Source: CAD feature listing. Evaluate the final solid. Frame: model axes, mm. A direction names the side the tool comes from. Give positions to 0.01 mm unless a question says otherwise; leave off trailing zeros. Order: outer loops, then holes, each group sorted by start corner. A loop starts at its lowest first (then second) coordinate and runs counter-clockwise, first axis right, second up.
```python
from build123d import *

# Parameters (mm, degrees)
F0_W      = 76.2
F0_H      = 76.2
F1_DEPTH  = 38.1
F2_W      = 11.73516
F2_H      = 2.54
F3_DEPTH  = 1.27
F5_DEPTH  = 1.27
F7_DEPTH  = 1.27
F9_DEPTH  = 1.27
F11_DEPTH = 1.27
F13_DEPTH = 1.27
F14_R     = 1.27


with BuildPart() as f1:
    # F0 (on Top) → F1 (new body, symmetric)
    with BuildSketch(Plane.XY):
        Rectangle(F0_W, F0_H)
    extrude(amount=F1_DEPTH, both=True)

    # F2 (on face) → F3 (cut, symmetric)
    with BuildSketch(Plane.XZ.offset(38.1)):
        with Locations((-7.13758, 21.63039)):
            Rectangle(F2_W, F2_H)
        Polygon((0, 22.90039), (-1.27, 22.90039), (-1.27, 20.36039), (0, 20.36039), (1.27, 20.36039), (1.27, 22.90039), align=None)
        Polygon((0, 20.36039), (-1.27, 20.36039), (-1.27, 0), (-1.27, -22.90039), (0, -22.90039), (1.27, -22.90039), (1.27, 0), (1.27, 20.36039), align=None)
        with Locations((7.13758, 21.63039)):
            Rectangle(F2_W, F2_H)
        Polygon((0, -22.90039), (-1.27, -22.90039), (-13.00516, -22.90039), (-13.00516, -25.44039), (0, -25.44039), (13.00516, -25.44039), (13.00516, -22.90039), (1.27, -22.90039), align=None)
    extrude(amount=F3_DEPTH, both=True, mode=Mode.SUBTRACT)

    # F4 (on face) → F5 (cut, symmetric)
    with BuildSketch(Plane(origin=(0, 38.1, 0), x_dir=(-1, 0, 0), z_dir=(0, 1, 0))):
        Polygon((5.588, 26.286197), (5.588, 23.746197), (10.960088, 23.746197), (12.230088, 23.746197), (13.500088, 23.746197), (19.957788, 23.746197), (19.957788, 26.286197), (12.230088, 26.286197), align=None)
        Polygon((12.230088, 23.746197), (10.960088, 23.746197), (10.960088, -21.1963), (12.230088, -21.1963), (13.500088, -21.1963), (13.500088, 23.746197), align=None)
        Polygon((12.230088, -21.1963), (10.960088, -21.1963), (5.588, -21.1963), (5.588, -23.7363), (12.230088, -23.7363), (19.957788, -23.7363), (19.957788, -21.1963), (13.500088, -21.1963), align=None)
        Polygon((-7.667548, 26.286197), (-14.804196, -10.425624), (-21.940843, 26.286197), (-24.528392, 26.286197), (-14.804196, -23.7363), (-5.08, 26.286197), align=None)
    extrude(amount=F5_DEPTH, both=True, mode=Mode.SUBTRACT)

    # F6 (on face) → F7 (cut, symmetric)
    with BuildSketch(Plane(origin=(-38.1, 0, 0), x_dir=(0, -1, 0), z_dir=(-1, 0, 0))):
        Polygon((-14.887291, 25.654), (0, -25.721655), (14.887291, 25.654), (12.2428, 25.654), (0, -16.595586), (-12.2428, 25.654), align=None)
    extrude(amount=F7_DEPTH, both=True, mode=Mode.SUBTRACT)

    # F8 (on face) → F9 (cut, symmetric)
    with BuildSketch(Plane.YZ.offset(38.1)):
        Polygon((-22.352, 27.513674), (-22.352, 24.973674), (-15.24, 24.973674), (-13.97, 24.973674), (-12.7, 24.973674), (-5.588, 24.973674), (-5.588, 27.513674), (-13.97, 27.513674), align=None)
        Polygon((-13.97, 24.973674), (-15.24, 24.973674), (-15.24, -26.48152), (-13.97, -26.48152), (-12.7, -26.48152), (-12.7, 24.973674), align=None)
        Polygon((-13.97, -26.48152), (-15.24, -26.48152), (-22.352, -26.48152), (-22.352, -29.02152), (-13.97, -29.02152), (-5.588, -29.02152), (-5.588, -26.48152), (-12.7, -26.48152), align=None)
        Polygon((13.97, 24.973674), (12.7, 24.973674), (12.7, -26.48152), (13.97, -26.48152), (15.24, -26.48152), (15.24, 24.973674), align=None)
        Polygon((5.588, 24.973674), (12.7, 24.973674), (13.97, 24.973674), (15.24, 24.973674), (22.352, 24.973674), (22.352, 27.513674), (13.97, 27.513674), (5.588, 27.513674), align=None)
        Polygon((13.97, -26.48152), (12.7, -26.48152), (5.588, -26.48152), (5.588, -29.02152), (13.97, -29.02152), (22.352, -29.02152), (22.352, -26.48152), (15.24, -26.48152), align=None)
    extrude(amount=F9_DEPTH, both=True, mode=Mode.SUBTRACT)

    # F10 (on face) → F11 (cut, symmetric)
    with BuildSketch(Plane(origin=(0, 0, -38.1), x_dir=(1, 0, 0), z_dir=(0, 0, -1))):
        Polygon((-22.352, 25.81735), (-22.352, 23.27735), (-15.24, 23.27735), (-13.97, 23.27735), (-12.7, 23.27735), (-5.588, 23.27735), (-5.588, 25.81735), (-13.97, 25.81735), align=None)
        Polygon((-13.97, 23.27735), (-15.24, 23.27735), (-15.24, -23.1902), (-13.97, -23.1902), (-12.7, -23.1902), (-12.7, 23.27735), align=None)
        Polygon((-13.97, -23.1902), (-15.24, -23.1902), (-22.352, -23.1902), (-22.352, -25.7302), (-13.97, -25.7302), (-5.588, -25.7302), (-5.588, -23.1902), (-12.7, -23.1902), align=None)
        Polygon((5.08, 25.81735), (16.829143, -25.7302), (28.578286, 25.81735), (25.973143, 25.81735), (16.829143, -14.300538), (7.685143, 25.81735), align=None)
    extrude(amount=F11_DEPTH, both=True, mode=Mode.SUBTRACT)

    # F12 (on face) → F13 (cut, symmetric)
    with BuildSketch(Plane.XY.offset(38.1)):
        Polygon((27.891114, -27.228153), (27.891114, -24.688153), (21.323074, -24.688153), (20.053074, -24.688153), (18.783074, -24.688153), (12.215033, -24.688153), (12.215033, -27.228153), (20.053074, -27.228153), align=None)
        Polygon((20.053074, -24.688153), (21.323074, -24.688153), (21.323074, 24.24637), (20.053074, 24.24637), (18.783074, 24.24637), (18.783074, -24.688153), align=None)
        Polygon((20.053074, 24.24637), (21.323074, 24.24637), (27.891114, 24.24637), (27.891114, 26.78637), (20.053074, 26.78637), (12.215033, 26.78637), (12.215033, 24.24637), (18.783074, 24.24637), align=None)
        Polygon((7.83804, -27.228153), (7.83804, -24.688153), (1.27, -24.688153), (0, -24.688153), (-1.27, -24.688153), (-7.83804, -24.688153), (-7.83804, -27.228153), (-0.004473, -27.228153), (0.004473, -27.228153), align=None)
        Polygon((0, -24.688153), (1.27, -24.688153), (1.27, 24.24637), (0, 24.24637), (-1.27, 24.24637), (-1.27, -24.688153), align=None)
        Polygon((0, 24.24637), (1.27, 24.24637), (7.83804, 24.24637), (7.83804, 26.78637), (0, 26.78637), (-7.83804, 26.78637), (-7.83804, 24.24637), (-1.27, 24.24637), align=None)
        Polygon((-20.053074, -27.228153), (-12.215033, -27.228153), (-12.215033, -24.688153), (-18.783074, -24.688153), (-20.053074, -24.688153), (-21.323074, -24.688153), (-27.891114, -24.688153), (-27.891114, -27.228153), align=None)
        Polygon((-20.053074, -24.688153), (-18.783074, -24.688153), (-18.783074, 24.24637), (-20.053074, 24.24637), (-21.323074, 24.24637), (-21.323074, -24.688153), align=None)
        Polygon((-20.053074, 24.24637), (-18.783074, 24.24637), (-12.215033, 24.24637), (-12.215033, 26.78637), (-20.053074, 26.78637), (-27.891114, 26.78637), (-27.891114, 24.24637), (-21.323074, 24.24637), align=None)
    extrude(amount=F13_DEPTH, both=True, mode=Mode.SUBTRACT)

    # F14
    f14_edges = [f1.edges().sort_by_distance(p)[0] for p in [
        (38.1, 0, 38.1),
        (0, -38.1, 38.1),
        (-38.1, 0, 38.1),
        (0, 38.1, 38.1),
        (-38.1, -38.1, 0),
        (0, -38.1, -38.1),
        (38.1, -38.1, 0),
        (-38.1, 0, -38.1),
        (-38.1, 38.1, 0),
        (38.1, 38.1, 0),
        (0, 38.1, -38.1),
        (38.1, 0, -38.1),
    ]]
    fillet(f14_edges, radius=F14_R)


solid = f1.part
```
1) Section query A-A, the plane x = 20. Return the cut outline in (y, z).
Report:
outline: (-38.1, -36.83) arc R1.27 ccw to (-36.83, -38.1) - (0.39, -38.1) - (0.39, -36.83) - (11.82, -36.83) - (11.82, -38.1) - (36.83, -38.1) arc R1.27 ccw to (38.1, -36.83) - (38.1, 2.99) - (36.83, 2.99) - (36.83, 16.3) - (38.1, 16.3) - (38.1, 36.83) arc R1.27 ccw to (36.83, 38.1) - (26.79, 38.1) - (26.79, 36.83) - (-27.23, 36.83) - (-27.23, 38.1) - (-36.83, 38.1) arc R1.27 ccw to (-38.1, 36.83) - close
2) Pin query (flat end, axial travel): pin 1 (1 mm diameter, centred on x = 37.5, z = -28, fed in from +Y); pin 2 (0.6 mm diameter, centred on x = -6, y = -37.5, fed in from +Z); pin 3 (1 mm diameter, centred on y = 1.5, z = 37.5, fed in from +X). Return the tip coordinate at first contact, or that it passes through.
Report:
pin 1: stops at y = 38.09
pin 2: stops at z = 38.04
pin 3: stops at x = 38.09
3) Material intervals for L1, parallel to Y at x = 12.5, z = -8, sorted ascending.
Report:
L1: y = -38.1 to 36.83
4) Reachability of faces 5 (the flat face through (-37.47, 7.55, 0.33)), 6 (the flat face through (12, -4, -36.83)), 7 (the flat face through (10.01, 37.47, 0.92)) from +Z, -Z, +X, -X, +Y, -Y: full face, straight path, thin tool, end or side. Return the list, or none.
Report:
face 5: -X
face 6: -Z
face 7: +Y
5) Draft query along Y for faces 1 (the flat face through (-1, 38.1, 1)), 2 (the flat face through (-21, 0, 36.83)), 3 (the flat face through (36.83, 15, -1)), 4 (the flat face through (-38.1, -1, 1)). Return one class per face: +Y half, -Y half, draft (parallel to the pull), parting line (faces both ways), or undercut.
Report:
face 1: +Y half
face 2: undercut
face 3: undercut
face 4: draft
